Check sheet for the modelled part. Datum: model origin and axes. Units: mm. Face numbers are marked on the shaded views. A direction names the side the tool comes from. Round coordinates to 2 decimals unless told otherwise and drop trailing zeros. Loops run counter-clockwise (first coordinate to the right, second up) from the corner with the lowest first, then second, coordinate; pieces in that order, holes last. Notation, with made-up numbers: (81.25, 17) - (98.25, 17) arc R14 cw to (98.25, 39) - close; hole circle Ø11 at (-17, -10.5). An arc over 180 degrees is marked (long way). Put each result on its own line as item: value. Start each with the question number.
Item 1: Gauge pin test, flat ends, axial feed: pin 1 Ø5.5 at (x, y) = (0.5, -11.5) entering from +Z; pin 2 Ø1.5 at (y, z) = (-18.5, 3.5) entering from +X; pin 3 Ø2.5 at (y, z) = (-19, 2.5) entering from -X; pin 4 Ø3 at (x, z) = (-0.5, 3.5) entering from +Y. Record the tip position at first contact, or that the pin passes through.
Item 2: Section check C-C, the plane z = 27. Record the cut outline in (x, y) (3 decimals).
Item 3: Tool access check on the marked faces 4, 5 and 6. Record the directions out of +Z, -Z, +X, -X, +Y, -Y that give a thin tool (end or side, any length) a straight path to the whole face; none if there is none.
Item 4: Section check B-B, the plane z = 14. Record the cut outline in (x, y) (3 decimals), and give its area (3 significant figures).
Item 5: Section check A-A, the plane x = 0. Record the cut outline in (y, z).
Item 6: Material ranges on line 1 along X through (y, z) = (-9, 9.5) (3 decimals); line 2 along Z through (x, y) = (-1.5, -4.5); line 3 along Z through (x, y) = (27.5, -10.9), recorded low to high.
Item 7: Draft check along X on the marked faces 1, 2 and 3. Enter one of: pulls with the +X half, pulls with the -X half, needs draft (parallel to the pull), parting line crosses it, or undercut.
Item 8: Section check D-D, the plane y = -1.5. Record the cut outline in (x, z) (3 decimals).
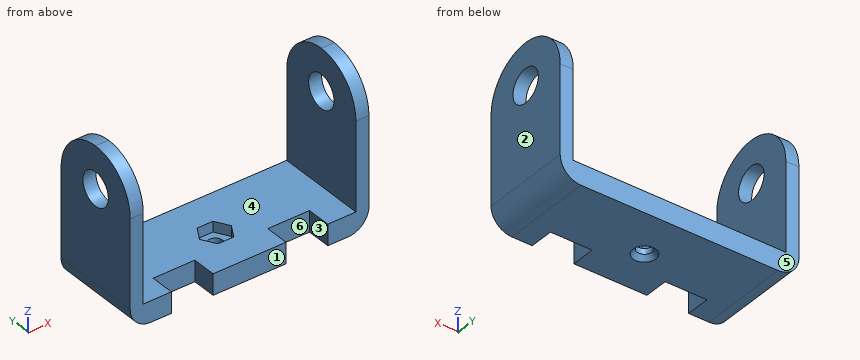
from build123d import *

# Parameters (mm, degrees)
F1_DEPTH       = 21.8
F2_R           = 4
F3_DEPTH       = 69.8
F4_R           = 10.89999
F5_W           = 10
F5_H           = 5.75
F5_H_2         = 0.9999994934
F6_DEPTH       = 25
F7_D           = 3.5
F7_DEPTH       = 10
F7_CSINK_D     = 5.5
F7_CSINK_ANGLE = 82
F7_TIP         = 1.0515060833
F8_R           = 1.75
F9_DEPTH       = 2.5
F10_R          = 5


# Not quite as in the source:
# - a fillet or chamfer is up to 0.001 mm smaller than in the source, because OpenCascade refuses the exact size


with BuildPart() as f1:
    # F0 (on Front) → F1 (new body)
    with BuildSketch(Plane.XZ):
        Polygon((-25.5, 37), (-28.625, 37), (-28.625, 0), (28.625, 0), (28.625, 37), (25.5, 37), (25.5, 5), (-25.5, 5), align=None)
    extrude(amount=F1_DEPTH)

    # F2 (on face) → F3 (cut)
    with BuildSketch(Plane(origin=(-28.625, 0, 0), x_dir=(0, -1, 0), z_dir=(-1, 0, 0))):
        with Locations((10.9, 27)):
            Circle(F2_R)
    extrude(amount=-F3_DEPTH, mode=Mode.SUBTRACT)

    # F4 (radius 10.9 in the source; OpenCascade refuses exactly that, so slightly less here)
    f4_edges = [f1.edges().sort_by_distance(p)[0] for p in [
        (-27.0625, -21.8, 37),
        (-27.0625, 0, 37),
        (27.0625, 0, 37),
        (27.0625, -21.8, 37),
    ]]
    fillet(f4_edges, radius=F4_R)

    # F5 (on face) → F6 (cut)
    with BuildSketch(Plane(origin=(0, 0, 0), x_dir=(1, 0, 0), z_dir=(0, 0, -1))):
        with Locations((-13.7500007451, 18.925)):
            Rectangle(F5_W, F5_H)
        with Locations((-13.7500007451, 22.2999997467)):
            Rectangle(F5_W, F5_H_2)
        with Locations((13.7500007451, 22.2999997467)):
            Rectangle(F5_W, F5_H_2)
        with Locations((13.7500007451, 18.925)):
            Rectangle(F5_W, F5_H)
    extrude(amount=-F6_DEPTH, mode=Mode.SUBTRACT)

    # F7
    with Locations(Plane(origin=(0, 0, 0), x_dir=(1, 0, 0), z_dir=(0, 0, -1))):
        with Locations((0, 11.05)):
            CounterSinkHole(F7_D / 2, F7_CSINK_D / 2, depth=F7_DEPTH, counter_sink_angle=F7_CSINK_ANGLE)
            with Locations((0, 0, -(F7_DEPTH + F7_TIP / 2))):  # 118° drill point
                Cone(0, F7_D / 2, F7_TIP, mode=Mode.SUBTRACT)

    # F8 (on face) → F9 (cut)
    with BuildSketch(Plane.XY.offset(5)):
        Polygon((1.9052558883, -7.75), (-1.9052558883, -7.75), (-3.8105117767, -11.05), (-1.9052558883, -14.35), (1.9052558883, -14.35), (3.8105117767, -11.05), align=None)
        with Locations((0, -11.05)):
            Circle(F8_R, mode=Mode.SUBTRACT)
    extrude(amount=-F9_DEPTH, mode=Mode.SUBTRACT)

    # F10
    f10_edges = [f1.edges().sort_by_distance(p)[0] for p in [
        (-28.625, -10.9, 0),
        (28.625, -10.9, 0),
    ]]
    fillet(f10_edges, radius=F10_R)


solid = f1.part
Check result:
1. pin 1: z = 5
1. pin 2: x = 28.57
1. pin 3: x = -28.47
1. pin 4: y = 0
2. outline: (-28.625, -21.763) - (-25.5, -21.763) - (-25.5, -14.9) - (-28.625, -14.9) - close; (-28.625, -6.9) - (-25.5, -6.9) - (-25.5, -0.037) - (-28.625, -0.037) - close; (25.5, -21.763) - (28.625, -21.763) - (28.625, -14.9) - (25.5, -14.9) - close; (25.5, -6.9) - (28.625, -6.9) - (28.625, -0.037) - (25.5, -0.037) - close
3. face 4: +Z, +Y, -Y
3. face 5: +Z, -Z, +X, -X, +Y
3. face 6: +Z, -Z, -Y
4. outline: (-28.625, -21.8) - (-25.5, -21.8) - (-25.5, 0) - (-28.625, 0) - close; (25.5, -21.8) - (28.625, -21.8) - (28.625, 0) - (25.5, 0) - close
4. area: 136 mm²
5. outline: (-21.8, 0) - (-13.8, 0) - (-12.8, 1.15) - (-12.8, 2.5) - (-14.35, 2.5) - (-14.35, 5) - (-21.8, 5) - close; (-9.3, 1.15) - (-8.3, 0) - (0, 0) - (0, 5) - (-7.75, 5) - (-7.75, 2.5) - (-9.3, 2.5) - close
6. line 1: -28.625 to -25.5, 25.5 to 28.625
6. line 2: 0 to 5
6. line 3: 1.84 to 23, 31 to 37
7. face 1: needs draft
7. face 2: pulls with the +X half
7. face 3: undercut
8. outline: (-28.625, 5) arc R5 ccw to (-23.625, 0) - (23.625, 0) arc R5 ccw to (28.625, 5) - (28.625, 31.618) - (25.5, 31.618) - (25.5, 5) - (-25.5, 5) - (-25.5, 31.618) - (-28.625, 31.618) - close
